Geometry: final body of the model. Coordinates: model frame, mm. A direction names the side the tool comes from. Round coordinates to 2 decimals unless told otherwise and drop trailing zeros. Loops run counter-clockwise (first coordinate to the right, second up) from the corner with the lowest first, then second, coordinate; pieces in that order, holes last. Notation, with made-up numbers: (64.5, 47.25) - (118.5, 47.25) arc R24 ccw to (118.5, 77.25) - close; hole circle Ø1 at (21, 75.25). An arc over 180 degrees is marked (long way). Answer as CSV lines item,"result".
from build123d import *

# Parameters (mm, degrees)
F1_DEPTH = 63.5
F2_DEPTH = 25.4
F3_DEPTH = 7.9375


with BuildPart() as f1:
    # F0 (on Front) → F1 (new body, symmetric)
    with BuildSketch(Plane.XZ):
        Polygon((44.9793039322, 9.525), (-18.5206960678, 9.525), (-18.5206960678, -9.525), (64.0293039322, -9.525), (64.0293039322, 9.525), align=None)
    extrude(amount=F1_DEPTH, both=True)

    # F0 (on Front) → F2 (join, symmetric)
    with BuildSketch(Plane.XZ):
        with BuildLine():
            Line((44.9793039322, 27.0002), (44.9793039322, 9.525))
            Line((44.9793039322, 9.525), (64.0293039322, 9.525))
            Line((64.0293039322, 9.525), (64.0293039322, 27.0002))
            ThreePointArc((64.0293039322, 27.0002), (68.6789837809, 38.2255201513), (79.9043039322, 42.8752))
            Line((79.9043039322, 42.8752), (83.0793039322, 42.8752))
            Line((83.0793039322, 42.8752), (83.0793039322, 61.9252))
            Line((83.0793039322, 61.9252), (79.9043039322, 61.9252))
            add(Edge.make_bspline(
                [(79.5426989751, 61.9233279649), (79.6630155752, 61.9240698804), (79.7835503929, 61.9246940115), (79.9043039322, 61.9252)],
                knots=[111.336027501, 111.336027501, 111.336027501, 111.336027501, 111.5045361635, 111.5045361635, 111.5045361635, 111.5045361635], degree=3))
            ThreePointArc((79.5426989751, 61.9233279649), (55.0810821618, 51.5677250267), (44.9793039322, 27.0002))
        make_face()
        Polygon((108.5640043465, 61.9252), (83.0793039322, 61.9252), (83.0793039322, 42.8752), (108.9037118903, 42.8752), align=None)
    extrude(amount=F2_DEPTH, both=True)

    # F0 (on Front) → F3 (join, symmetric)
    with BuildSketch(Plane.XZ):
        with BuildLine():
            add(Edge.make_bspline(
                [(-18.5206960678, 9.525), (15.8143353949, 9.525), (0.0478403981, 61.4331340424), (79.5426989751, 61.9233279649)],
                knots=[0, 0, 0, 0, 111.336027501, 111.336027501, 111.336027501, 111.336027501], degree=3))
            Line((-18.5206960678, 9.525), (44.9793039322, 9.525))
            Line((44.9793039322, 9.525), (44.9793039322, 27.0002))
            ThreePointArc((44.9793039322, 27.0002), (55.0810821618, 51.5677250267), (79.5426989751, 61.9233279649))
        make_face()
    extrude(amount=F3_DEPTH, both=True)

    # F0 (on Front) → F4 (revolve)
    with BuildSketch(Plane.XZ):
        Polygon((108.4793039322, 66.675), (108.5640043465, 61.9252), (108.9037118903, 42.8752), (109.0454831719, 34.925), (133.8793039322, 34.925), (133.8793039322, 66.675), align=None)
    revolve(axis=Axis((108.7623935521, 0, 50.8), (0.0178295824, 0, -0.9998410404)))


solid = f1.part
(1) Access query for faces 5 (the face through (44.979, 17, 18)), 6 (the face through (69, -25.4, 42)), 7 (the face through (83.6, -2, 42.875)), 8 (the face through (69, 25.4, 42)). Directions: +Z, -Z, +X, -X, +Y, -Y. A direction counts if a zero-diameter tool reaches every point of the face in a straight line with its end or side. Return the directions, or none.
Findings below:
face 5,"+Z, -X, +Y"
face 6,"+Z, +X, -X, -Y"
face 7,"-Z"
face 8,"+Z, +X, -X, +Y"
(2) Pin query (flat end, axial travel): P1, Ø16.5, axis at x = 20.5, y = 41.5, coming from the +Z side (3 decimals); P2, Ø14.5, axis at x = 99, y = 1.5, coming from the -Z side; P3, Ø6, axis at x = 29.5, z = 22, coming from the +Y side. Return the tip coordinate at first contact, or that it passes through.
Findings below:
P1,"z = 9.525"
P2,"z = 34.31"
P3,"y = 7.94"
(3) Section A-A (y = 30). Output: boundary loops of the cut face in (x, z) (3 decimals).
Findings below:
outline,"(-18.521, -9.525) - (64.029, -9.525) - (64.029, 9.525) - (-18.521, 9.525) - close"
(4) Draft query along Y for faces 1 (the face through (31, 7.938, 32)), 2 (the face through (64.029, -1, 4)), 3 (the face through (22, -63.5, 0)), 4 (the face through (110.481, 0.595, 34.923)). Return one class per face: pulls with the +Y half, pulls with the -Y half, needs draft (parallel to the pull), parting line crosses it, or undercut.
Findings below:
face 1,"pulls with the +Y half"
face 2,"needs draft"
face 3,"pulls with the -Y half"
face 4,"undercut"
(5) Material intervals for line 1 along Z through (x, y) = (28.5, 31) (3 decimals); line 2 along Y through (x, z) = (51.5, 38.5); line 3 along X through (y, z) = (18.5, 14), sorted ascending.
Findings below:
line 1,"-9.525 to 9.525"
line 2,"-25.4 to 25.4"
line 3,"44.98 to 64.03"
